Read the model definition and answer for the solid it produces. Units are mm, in the model's axes. A direction names the side the tool comes from. Round coordinates to 2 decimals unless told otherwise and drop trailing zeros. Order: outer loops, then holes, each group sorted by start corner. A loop starts at its lowest first (then second) coordinate and runs counter-clockwise, first axis right, second up. Notation, with made-up numbers: (2.25, -32) -> (61.25, -32) arc R9 cw to (61.25, -19) -> close; hole circle Ø10 at (86.5, 29). An arc over 180 degrees is marked (long way). Use a Markdown table: item, result. Add a question column.
1. Given pin 1 (2 mm diameter, centred on x = -5.5, z = -8, fed in from +Y); pin 2 (2 mm diameter, centred on x = 14.5, z = -18.5, fed in from +Y); pin 3 (5 mm diameter, centred on y = -13.5, z = 23.5, fed in from -X), each flat-ended and moving along its own axis, determine where each tip first touches the part or whether it passes through.
2. For faces 4 (the face through (28.996, 49, -37)), 5 (the face through (13.38, -25.725, 0.644)), 6 (the face through (-0.638, 124.673, -36.958)), determine the directions among +Z, -Z, +X, -X, +Y, -Y from which every point of the face is accessible in a straight line to the end or side of a thin tool.
3. The mould has two halves that part along X. Classify faces 1 (the face through (0.638, 125.524, 36.457)), 2 (the face through (-28.996, 49, 36)), 3 (the face through (-2.487, -11.197, -0.644)): +X half, -X half, draft (parallel to the pull), parting line (faces both ways), or undercut.
4. Section C-C, the plane x = 0 is taken. Give the vertices of the cut face in (y, z), then the cut area to 3 significant figures.
5. Section A-A, the plane y = 51.5 is taken. Give the vertices of the cut face in (x, z).
6. Section B-B, the plane z = -32 is taken. Give the vertices of the cut face in (x, y), then the cut area to 3 significant figures.
7. Section D-D, the plane y = 20 is taken. Give the vertices of the cut face in (x, z), then the cut area to 3 significant figures.
8. Consider L1, parallel to Z at x = -20.5, y = 53.5; L2, parallel to Y at x = 8, z = -28; L3, parallel to Y at x = 1.5, z = -36. Determine where each line is inside the solid, lowest interval first. Write a range as [from, to].
```python
from build123d import *

# Parameters (mm, degrees)
F0_R     = 28.9961675247
F0_R_2   = 11.4701678976
F1_DEPTH = 45.974
F3_DEPTH = 19.304
F5_DEPTH = 18.288


# Not quite as in the source:
# - ends of sketch curves that miss each other by under 0.0002 mm in the source are joined


with BuildPart() as f1:
    # F0 (on Top) → F1 (new body, symmetric)
    with BuildSketch(Plane.XY):
        Circle(F0_R)
        Circle(F0_R_2, mode=Mode.SUBTRACT)
    extrude(amount=F1_DEPTH, both=True)

    # F2 (on face) → F3 (join)
    with BuildSketch(Plane.XY.offset(45.974)):
        with BuildLine():
            ThreePointArc((-28.9961675247, 96.5353175998), (0, 67.5391500751), (28.9961675247, 96.5353175998))
            ThreePointArc((28.9961675247, 96.5353175998), (0, 125.5314851244), (-28.9961675247, 96.5353175998))
        make_face()
        with BuildLine():
            ThreePointArc((-13.7561708689, 96.5353175998), (0, 110.2914884686), (13.7561708689, 96.5353175998))
            ThreePointArc((13.7561708689, 96.5353175998), (0, 82.7791500751), (-13.7561708689, 96.5353175998))
        make_face(mode=Mode.SUBTRACT)
        with BuildLine():
            Line((-28.9961675247, 96.5353175998), (-28.9961675247, 0))
            ThreePointArc((-28.9961675247, 0), (0, 28.9961675247), (28.9961675247, 0))
            Line((28.9961675247, 0), (28.9961675247, 96.5353175998))
            ThreePointArc((28.9961675247, 96.5353175998), (0, 67.5391500751), (-28.9961675247, 96.5353175998))
        make_face()
    extrude(amount=-F3_DEPTH)

    # F4 (on face) → F5 (join)
    with BuildSketch(Plane(origin=(0, 0, -45.974), x_dir=(1, 0, 0), z_dir=(0, 0, -1))):
        with BuildLine():
            Line((28.9961675247, -95.6837162375), (28.9961675247, 0))
            ThreePointArc((28.9961675247, 0), (0, -28.9961675247), (-28.9961675247, 0))
            Line((-28.9961675247, 0), (-28.9961675247, -95.6837162375))
            ThreePointArc((-28.9961675247, -95.6837162375), (0, -66.6875487129), (28.9961675247, -95.6837162375))
        make_face()
        with BuildLine():
            ThreePointArc((-28.9961675247, -95.6837162375), (0, -124.6798837622), (28.9961675247, -95.6837162375))
            ThreePointArc((28.9961675247, -95.6837162375), (0, -66.6875487129), (-28.9961675247, -95.6837162375))
        make_face()
        with BuildLine():
            ThreePointArc((14.2641663551, -95.6837162375), (0, -109.9478825927), (-14.2641663551, -95.6837162375))
            ThreePointArc((-14.2641663551, -95.6837162375), (0, -81.4195498824), (14.2641663551, -95.6837162375))
        make_face(mode=Mode.SUBTRACT)
    extrude(amount=-F5_DEPTH)


solid = f1.part
```
Verdict:
| question | item | result |
|---|---|---|
| 1 | pin 1 | stops at y = 28.64 |
| 1 | pin 2 | stops at y = 25.66 |
| 1 | pin 3 | stops at x = -26.83 |
| 2 | face 4 | +Z, -Z, +X, +Y, -Y |
| 2 | face 5 | none |
| 2 | face 6 | -Z, +Y |
| 3 | face 1 | parting line |
| 3 | face 2 | -X half |
| 3 | face 3 | undercut |
| 4 | outline | (-29, -45.97) -> (-11.47, -45.97) -> (-11.47, 45.97) -> (-29, 45.97) -> close; (11.47, -45.97) -> (81.42, -45.97) -> (81.42, -27.69) -> (29, -27.69) -> (29, 26.67) -> (82.78, 26.67) -> (82.78, 45.97) -> (11.47, 45.97) -> close; (109.95, -45.97) -> (124.68, -45.97) -> (124.68, -27.69) -> (109.95, -27.69) -> close; (110.29, 26.67) -> (125.53, 26.67) -> (125.53, 45.97) -> (110.29, 45.97) -> close |
| 4 | area | 5,780 mm2 |
| 5 | outline | (-29, -45.97) -> (29, -45.97) -> (29, -27.69) -> (-29, -27.69) -> close; (-29, 26.67) -> (29, 26.67) -> (29, 45.97) -> (-29, 45.97) -> close |
| 6 | outline | (-29, 0) arc R29 ccw to (29, 0) -> (29, 95.68) arc R29 ccw to (-29, 95.68) -> close; hole circle Ø28.53 at (0, 95.68); hole circle Ø22.94 at (0, 0) |
| 6 | area | 7,140 mm2 |
| 7 | outline | (-29, -45.97) -> (29, -45.97) -> (29, -27.69) -> (20.99, -27.69) -> (20.99, 26.67) -> (29, 26.67) -> (29, 45.97) -> (-29, 45.97) -> (-29, 26.67) -> (-20.99, 26.67) -> (-20.99, -27.69) -> (-29, -27.69) -> close |
| 7 | area | 4,460 mm2 |
| 8 | L1 | z = [-45.97, -27.69], [26.67, 45.97] |
| 8 | L2 | y = [-27.87, -8.22], [8.22, 83.87], [107.49, 123.55] |
| 8 | L3 | y = [-28.96, -11.37], [11.37, 81.5], [109.87, 124.64] |
